Check sheet for the drawn part. Datum: minimum x, y, z corner. Units: mm. A direction names the side the tool comes from. Coordinates: 2 decimals unless noted, no trailing zeros. Order: outer loops, then holes, each group sorted by start corner. A loop starts at its lowest first (then second) coordinate and runs counter-clockwise, first axis right, second up. Notation, with made-up numbers: (62, -0.5) - (112, -0.5) arc R34 cw to (112, 36.5) - close; hole circle Ø11 at (16, -38.75). An arc over 180 degrees is marked (long way). One line per item, written item: value. Start each with the question number.
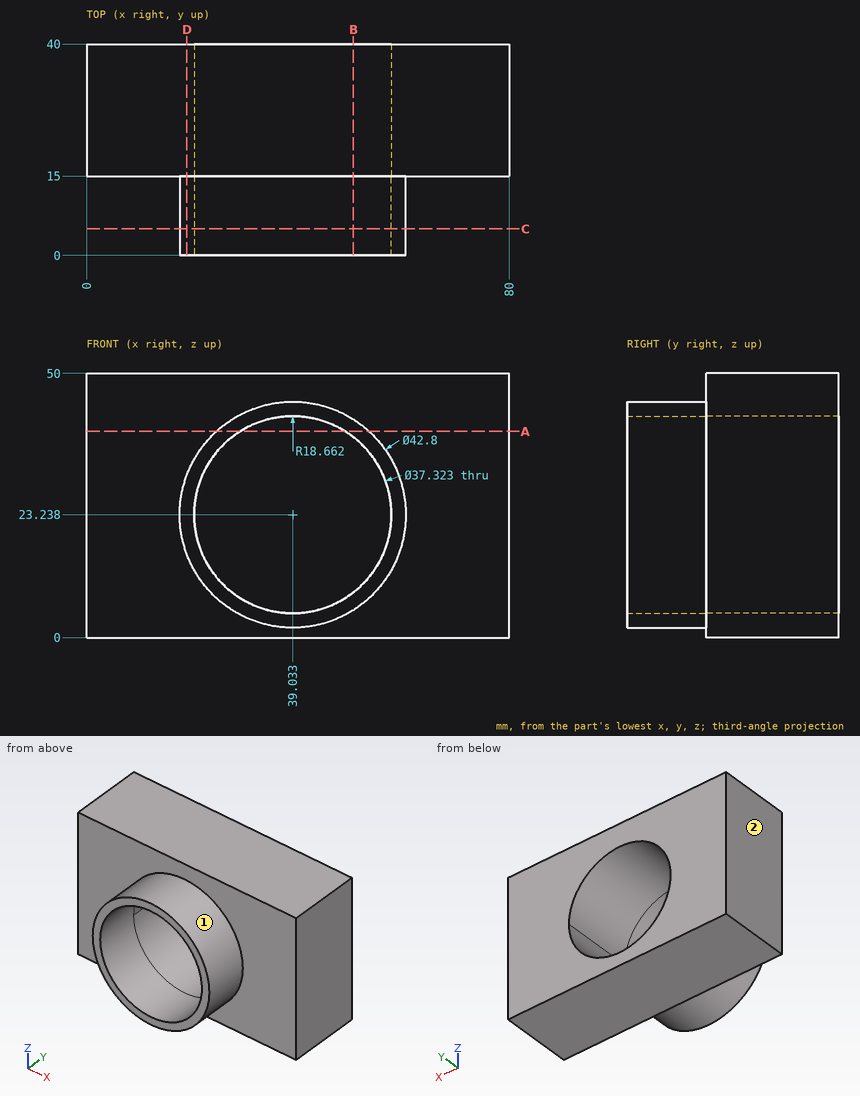
Q1. Cross-section at C-C, the plane y = 5. Enter the section's corners in (x, z).
Q2. Gauge pin test, flat ends, axial feed: P1, Ø1, axis at x = 62.5, y = 16.5, coming from the -Z side; P2, Ø5, axis at y = 5.5, z = 45, coming from the -X side (1 decimal); P3, Ø1, axis at x = 33, y = 13.5, coming from the +Z side. Record the tip position at first contact, or that the pin passes through.
Q3. Material ranges on probe 1 along Y at (x, z) = (59, 14.5); probe 2 along X at (y, z) = (17, 31.5) (1 decimal); probe 3 along Z at (x, y) = (22, 4) (1 decimal), recorded low to high.
Q4. Cross-section at A-A, the plane z = 39. Enter the section's corners in (x, y).
Q5. Set-up check for the marked faces 1 and 2: record each of +Z, -Z, +X, -X, +Y, -Y from which the full face is reachable in a straight line by a thin tool's end or side.
Q6. Cross-section at D-D, the plane x = 19. Enter the section's corners in (y, z) (1 decimal), and give its area (3 significant figures).
Q7. Cross-section at B-B, the plane x = 50.5. Enter the section's corners in (y, z) (1 decimal).
Check result:
1. outline: circle Ø42.8 at (39.03, 23.24); hole circle Ø37.32 at (39.03, 23.24)
2. P1: stops at z = 0
2. P2: stops at x = 29.7
2. P3: stops at z = 43.91
3. probe 1: y = 15 to 40
3. probe 2: x = 0 to 22.3, 55.8 to 80
3. probe 3: z = 10.3 to 15.6, 30.9 to 36.2
4. outline: (0, 15) - (24.56, 15) - (24.56, 0) - (29.04, 0) - (29.04, 40) - (0, 40) - close; (49.02, 0) - (53.51, 0) - (53.51, 15) - (80, 15) - (80, 40) - (49.02, 40) - close
5. face 1: -Y
5. face 2: +Z, -Z, -X, +Y, -Y
6. outline: (0, 15.7) - (15, 15.7) - (15, 0) - (40, 0) - (40, 50) - (15, 50) - (15, 30.8) - (0, 30.8) - close
6. area: 1,480 mm2
7. outline: (0, 5.2) - (15, 5.2) - (15, 0) - (40, 0) - (40, 8.5) - (0, 8.5) - close; (0, 38) - (40, 38) - (40, 50) - (15, 50) - (15, 41.3) - (0, 41.3) - close
